from build123d import *

# Parameters (mm, degrees)
SKETCH1_W                   = 100
SKETCH1_H                   = 50
SKETCH1_R                   = 0.5
BOSS_EXTRUDE6_DEPTH         = 10
SKETCH3_W                   = 100
SKETCH3_H                   = 50
BOSS_EXTRUDE7_DEPTH         = 10
M2_TAPPED_HOLE1_D           = 1.6
M2_TAPPED_HOLE1_DEPTH       = 20
M2_TAPPED_HOLE1_CSINK_D     = 2.05
M2_TAPPED_HOLE1_CSINK_ANGLE = 90
M2_TAPPED_HOLE1_TIP         = 0.480688495


with BuildPart() as part:
    # Sketch1 → Boss-Extrude6 (new body)
    with BuildSketch(Plane(origin=(0, 0, 0), x_dir=(1, 0, 0), z_dir=(0, 1, 0))):
        Rectangle(SKETCH1_W, SKETCH1_H)
        with Locations((-14.2, -7)):
            Circle(SKETCH1_R, mode=Mode.SUBTRACT)
        with Locations((14.2, -7)):
            Circle(SKETCH1_R, mode=Mode.SUBTRACT)
        with Locations((-16.685084167, 3.643524774)):
            Circle(SKETCH1_R, mode=Mode.SUBTRACT)
        with Locations((16.685084167, 3.643524774)):
            Circle(SKETCH1_R, mode=Mode.SUBTRACT)
        with Locations((-11.935084167, 5)):
            Circle(SKETCH1_R, mode=Mode.SUBTRACT)
        with Locations((11.935084167, 5)):
            Circle(SKETCH1_R, mode=Mode.SUBTRACT)
        Polygon((-11.7, 3), (-0.25, 3), (-0.25, 7), (0.25, 7), (0.25, 3), (11.7, 3), (11.7, -3), (-11.7, -3), align=None, mode=Mode.SUBTRACT)
    extrude(amount=BOSS_EXTRUDE6_DEPTH)

    # Sketch3 → Boss-Extrude7 (add)
    with BuildSketch(Plane(origin=(0, 10, 0), x_dir=(1, 0, 0), z_dir=(0, 1, 0))):
        Rectangle(SKETCH3_W, SKETCH3_H)
    extrude(amount=BOSS_EXTRUDE7_DEPTH)

    # M2 Tapped Hole1
    with Locations(Plane(origin=(0, 20, 0), x_dir=(1, 0, 0), z_dir=(0, 1, 0))):
        with Locations((-16.685084167, 3.643524774), (-11.935084167, 5), (11.935084167, 5), (16.685084167, 3.643524774), (14.2, -7), (-14.2, -7), (-8, 0), (8.042631754, 0), (0, 0)):
            CounterSinkHole(M2_TAPPED_HOLE1_D / 2, M2_TAPPED_HOLE1_CSINK_D / 2, depth=M2_TAPPED_HOLE1_DEPTH, counter_sink_angle=M2_TAPPED_HOLE1_CSINK_ANGLE)
            with Locations((0, 0, -(M2_TAPPED_HOLE1_DEPTH + M2_TAPPED_HOLE1_TIP / 2))):  # 118° drill point
                Cone(0, M2_TAPPED_HOLE1_D / 2, M2_TAPPED_HOLE1_TIP, mode=Mode.SUBTRACT)


solid = part.part
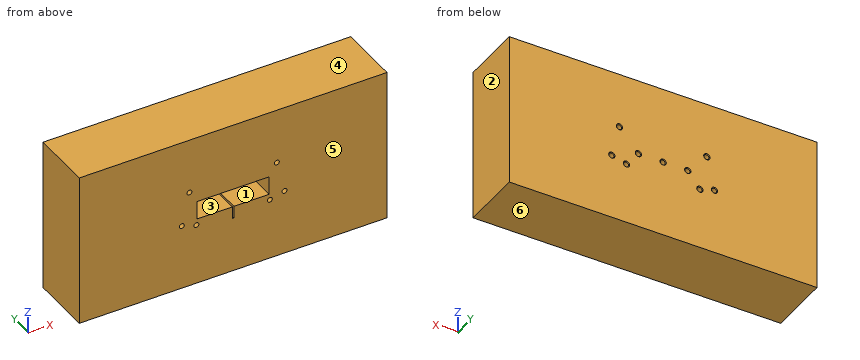
Work out the finished part from the listing and answer in its coordinate system (mm). Face numbers are marked on the shaded views. A direction names the side the tool comes from. Give positions to 0.01 mm unless a question says otherwise; leave off trailing zeros. Order: outer loops, then holes, each group sorted by start corner. A loop starts at its lowest first (then second) coordinate and runs counter-clockwise, first axis right, second up. Notation, with made-up numbers: (32, -26.75) -> (87, -26.75) arc R15 ccw to (87, 1.25) -> close; hole circle Ø10 at (11.5, -18). An arc over 180 degrees is marked (long way). One line per item, written item: value.
Item 1: A tool of negligible diameter and unlimited length cuts with its end or side. For the marked faces 1 and 2, from which of +Z, -Z, +X, -X, +Y, -Y can it reach the whole face along a straight path? Write none if from no direction.
Answer sheet:
face 1: -Y
face 2: +Z, -Z, +X, +Y, -Y
Item 2: Determine the mould class of the marked faces 3, 4, 5 and 6 for opening direction Z: released by +Z, released by -Z, zero draft, split by the parting line, or undercut.
Answer sheet:
face 3: undercut
face 4: released by +Z
face 5: zero draft
face 6: released by -Z
Item 3: Straight lines are drawn through the part: probe 1 along Z at (x, y) = (-14.2, 12.5); probe 2 along Z at (x, y) = (6.5, 6.5); probe 3 along Y at (x, z) = (7, -0.5). For each, find the intervals that lie inside material, in ascending order.
Answer sheet:
probe 1: -25 to 6.2, 7.8 to 25
probe 2: -25 to -3, 3 to 25
probe 3: 10 to 20
Item 4: Find section A-A, the plane y = 5.25. Give the vertices of the cut face in (x, z).
Answer sheet:
outline: (-50, -25) -> (50, -25) -> (50, 25) -> (-50, 25) -> close; hole circle Ø1.6 at (-16.69, -3.64); hole circle Ø1.6 at (-14.2, 7); hole circle Ø1.6 at (-11.94, -5); hole (-11.7, -3) -> (-0.25, -3) -> (-0.25, -7) -> (0.25, -7) -> (0.25, -3) -> (11.7, -3) -> (11.7, 3) -> (-11.7, 3) -> close; hole circle Ø1.6 at (11.94, -5); hole circle Ø1.6 at (14.2, 7); hole circle Ø1.6 at (16.69, -3.64)
